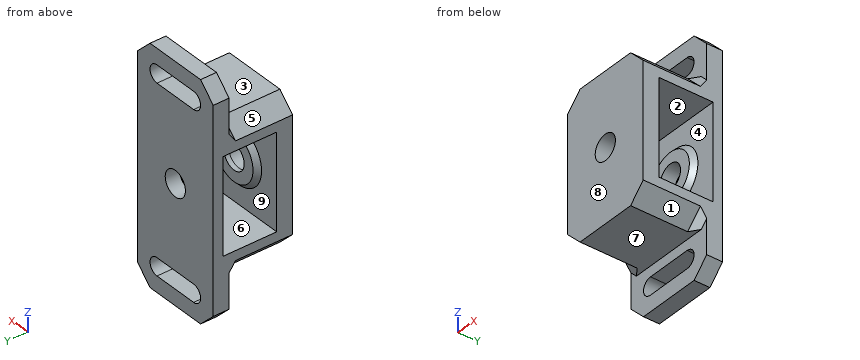
from build123d import *

# Parameters (mm, degrees)
F0_R     = 11
F0_R_2   = 4
F1_DEPTH = 3
F0_W     = 30
F0_H     = 8
F2_DEPTH = 20
F3_DEPTH = 5
F4_W     = 30
F4_H     = 46
F4_R     = 4
F5_DEPTH = 5
F6_R     = 7
F6_R_2   = 4
F7_DEPTH = 1.5
F8_R     = 7
F8_R_2   = 4
F9_DEPTH = 1.5
F10_SIZE = 5
F12_SIZE = 2


# Not quite as in the source:
# - a fillet or chamfer that OpenCascade refuses, or shapes differently, is made with other operations: its cross-section is extruded or revolved along the edge and cut away or added


with BuildPart() as f1:
    # F0 (on Front) → F1 (new body)
    with BuildSketch(Plane.XZ):
        Polygon((15, 15), (-15, 15), (-15, 0), (-15, -15), (15, -15), (15, 0), align=None)
        Circle(F0_R, mode=Mode.SUBTRACT)
        Circle(F0_R)
        Circle(F0_R_2, mode=Mode.SUBTRACT)
    extrude(amount=F1_DEPTH)

    # F0 (on Front) → F2 (join)
    with BuildSketch(Plane.XZ):
        with Locations((0, 19)):
            Rectangle(F0_W, F0_H)
        with Locations((0, -19)):
            Rectangle(F0_W, F0_H)
    extrude(amount=F2_DEPTH)

    # F0 (on Front) → F3 (join)
    with BuildSketch(Plane.XZ):
        Polygon((15, -23), (-15, -23), (-15, -36.75), (0, -36.75), (15, -36.75), align=None)
        with BuildLine():
            ThreePointArc((-7.25, -31.75), (-10, -29), (-7.25, -26.25))
            Line((-7.25, -26.25), (7.25, -26.25))
            ThreePointArc((7.25, -26.25), (10, -29), (7.25, -31.75))
            Line((7.25, -31.75), (-7.25, -31.75))
        make_face(mode=Mode.SUBTRACT)
        Polygon((-15, 36.75), (-15, 23), (15, 23), (15, 36.75), (0, 36.75), align=None)
        with BuildLine():
            ThreePointArc((-7.25, 26.25), (-10, 29), (-7.25, 31.75))
            Line((-7.25, 31.75), (7.25, 31.75))
            ThreePointArc((7.25, 31.75), (10, 29), (7.25, 26.25))
            Line((7.25, 26.25), (-7.25, 26.25))
        make_face(mode=Mode.SUBTRACT)
    extrude(amount=F3_DEPTH)

    # F4 (on face) → F5 (join)
    with BuildSketch(Plane.XZ.offset(20)):
        Rectangle(F4_W, F4_H)
        Circle(F4_R, mode=Mode.SUBTRACT)
    extrude(amount=F5_DEPTH)

    # F6 (on face) → F7 (join)
    with BuildSketch(Plane.XZ.offset(3)):
        Circle(F6_R)
        Circle(F6_R_2, mode=Mode.SUBTRACT)
    extrude(amount=F7_DEPTH)

    # F8 (on face) → F9 (join)
    with BuildSketch(Plane(origin=(0, -20, 0), x_dir=(-1, 0, 0), z_dir=(0, 1, 0))):
        Circle(F8_R)
        Circle(F8_R_2, mode=Mode.SUBTRACT)
    extrude(amount=F9_DEPTH)

    # F10
    f10_edges = [f1.edges().sort_by_distance(p)[0] for p in [
        (15, -2.5, 36.75),
        (-15, -2.5, 36.75),
        (15, -2.5, -36.75),
        (-15, -2.5, -36.75),
        (-15, -15, 23),
        (15, -15, 23),
        (15, -15, -23),
        (-15, -15, -23),
    ]]
    chamfer(f10_edges, length=F10_SIZE)

    # F11: chamfer of 2 on 2 edges, made by hand


with BuildPart() as f11_tool2:
    # F11_s3 → F11_t4 (revolve)
    with BuildSketch(Plane.XY):
        Polygon((9, -3), (7, -5), (7, -3), align=None)
    revolve(axis=Axis((0, -3, 0), (0, -1, 0)))

    split(bisect_by=Plane.XZ.offset(4.5), keep=Keep.BOTTOM)


with BuildPart() as f1_1:
    add(f1.part)

    # F11_t1: union F11_tool2
    add(f11_tool2.part)


with BuildPart() as f11_tool7:
    # F11_s8 → F11_t9 (revolve)
    with BuildSketch(Plane.XY):
        Polygon((-9, -20), (-7, -18), (-7, -20), align=None)
    revolve(axis=Axis((0, -20, 0), (0, 1, 0)))

    split(bisect_by=Plane.XZ.offset(18.5), keep=Keep.TOP)


with BuildPart() as f1_2:
    add(f1_1.part)

    # F11_t6: union F11_tool7
    add(f11_tool7.part)

    # F12
    f12_edges = [f1_2.edges().sort_by_distance(p)[0] for p in [
        (12.5, -5, 20.5),
        (-12.5, -5, 20.5),
        (-12.5, -5, -20.5),
        (12.5, -5, -20.5),
    ]]
    chamfer(f12_edges, length=F12_SIZE)


solid = f1_2.part
Here's how the part is built. I have some questions about the finished solid (model axes, mm). Face numbers are marked on the shaded views. A direction names the side the tool comes from. Give positions to 0.01 mm unless a question says otherwise; leave off trailing zeros. Order: outer loops, then holes, each group sorted by start corner. A loop starts at its lowest first (then second) coordinate and runs counter-clockwise, first axis right, second up. Notation, with made-up numbers: (57.5, 62) -> (110.5, 62) arc R27 ccw to (110.5, 80) -> close; hole circle Ø6 at (37.25, -21.5). An arc over 180 degrees is marked (long way). Use a Markdown table: item, result. Add a question column.
Item 1: Imagine slicing it at A-A on z = 0. Please give me the cut outline in (x, y), plus the area to 4 significant figures.
Item 2: Imagine slicing it at B-B on y = -10.5. Please give me the cut outline in (x, z), plus the area to 3 significant figures.
Item 3: Imagine slicing it at D-D on x = 0. Give the number of separate pieces and of enclosed holes in the cut face, plus the area to 3 significant figures.
Item 4: I need wall thicknesses on line 1 (Z direction, x = 0, y = -2.15); line 2 (Y direction, x = 2, z = -3.5); line 3 (Z direction, x = 1, y = -16). Which ranges of each line are inside material? Lowest first, please.
Item 5: For the marked faces 1, 2, 3, 4 and 5, which set-ups out of +Z, -Z, +X, -X, +Y, -Y let a thin tool reach every point of the face, with its end or its side?
Item 6: If we mould it in two halves opening along Z, with no side actions, what happens to the marked faces 6, 7, 8 and 9? For each: pulls with the +Z half, pulls with the -Z half, needs draft (parallel to the pull), parting line crosses it, or undercut.
Item 7: Imagine slicing it at C-C on z = -29. Please give me the cut outline in (x, y), plus the area to 3 significant figures.
Item 8: Will these pins go through, and if not, where does the flat tip stop? pin 1 (6 mm diameter, centred on x = 1, y = -10, fed in from +Z); pin 2 (5 mm diameter, centred on x = 1, z = -30.5, fed in from -Y); pin 3 (6 mm diameter, centred on x = -4, y = -8.5, fed in from -Z).
Data:
| question | item | result |
|---|---|---|
| 1 | outline | (-15, -25) -> (-4, -25) -> (-4, -18.5) -> (-7.5, -18.5) -> (-9, -20) -> (-15, -20) -> close; (-15, -3) -> (-9, -3) -> (-7.5, -4.5) -> (-4, -4.5) -> (-4, 0) -> (-15, 0) -> close; (4, -25) -> (15, -25) -> (15, -20) -> (9, -20) -> (7.5, -18.5) -> (4, -18.5) -> close; (4, -4.5) -> (7.5, -4.5) -> (9, -3) -> (15, -3) -> (15, 0) -> (4, 0) -> close |
| 1 | area | 201.5 mm² |
| 2 | outline | (-15, -18) -> (-10, -23) -> (10, -23) -> (15, -18) -> (15, -15) -> (-15, -15) -> close; (-15, 15) -> (15, 15) -> (15, 18) -> (10, 23) -> (-10, 23) -> (-15, 18) -> close |
| 2 | area | 430 mm² |
| 3 | separate pieces | 4 |
| 3 | enclosed holes | 0 |
| 3 | area | 684 mm² |
| 4 | line 1 | z = -36.75 to -31.75, -26.25 to -4, 4 to 26.25, 31.75 to 36.75 |
| 4 | line 2 | y = -25 to -18.5, -4.5 to 0 |
| 4 | line 3 | z = -23 to -15, 15 to 23 |
| 5 | face 1 | -Z, +X, -Y |
| 5 | face 2 | +X, -X |
| 5 | face 3 | +Z, +X, -X, -Y |
| 5 | face 4 | none |
| 5 | face 5 | +Z, -X, -Y |
| 6 | face 6 | undercut |
| 6 | face 7 | pulls with the -Z half |
| 6 | face 8 | needs draft |
| 6 | face 9 | undercut |
| 7 | outline | (-15, -5) -> (-10, -5) -> (-10, 0) -> (-15, 0) -> close; (10, -5) -> (15, -5) -> (15, 0) -> (10, 0) -> close |
| 7 | area | 50.0 mm² |
| 8 | pin 1 | stops at z = 23 |
| 8 | pin 2 | stops at y = -5 |
| 8 | pin 3 | stops at z = -23 |
